Design review of the part built by this model. Coordinates are the model's own, in mm. Face numbers are marked on the shaded views. Coordinates: 2 decimals unless noted, no trailing zeros. Loops run counter-clockwise (first coordinate to the right, second up) from the corner with the lowest first, then second, coordinate; pieces in that order, holes last. Notation, with made-up numbers: M 33.5,19.5 L 79.5,19.5 A15 ccw 79.5,30.5 Z; hole C -22,-5 d7. An arc over 180 degrees is marked long. Write item = value, one per line. Start each with the question number.
```python
from build123d import *

# Parameters (mm, degrees)
SKETCH1_R                            = 5.08
BOSS_EXTRUDE1_DEPTH                  = 88.9
TAPPED_HOLE_FOR_4_40_HELICOIL1_D     = 3.048
TAPPED_HOLE_FOR_4_40_HELICOIL1_DEPTH = 8.128
TAPPED_HOLE_FOR_4_40_HELICOIL1_TIP   = 0.915711583
TAPPED_HOLE_FOR_4_40_HELICOIL2_D     = 3.048
TAPPED_HOLE_FOR_4_40_HELICOIL2_DEPTH = 8.128
TAPPED_HOLE_FOR_4_40_HELICOIL2_TIP   = 0.915711583
CUT_EXTRUDE1_DEPTH                   = 6.08
CUT_EXTRUDE1_DEPTH_BACK              = 6.08
TAPPED_HOLE_FOR_4_40_HELICOIL3_D     = 3.048


with BuildPart() as part:
    # Sketch1 → Boss-Extrude1 (new body)
    with BuildSketch(Plane(origin=(0, 0, 0), x_dir=(1, 0, 0), z_dir=(0, 1, 0))):
        Circle(SKETCH1_R)
    extrude(amount=BOSS_EXTRUDE1_DEPTH)

    # Tapped Hole for #4-40 Helicoil1
    with Locations(Plane(origin=(0, 88.9, 0), x_dir=(1, 0, 0), z_dir=(0, 1, 0))):
        with Locations((0, 0)):
            Hole(TAPPED_HOLE_FOR_4_40_HELICOIL1_D / 2, depth=TAPPED_HOLE_FOR_4_40_HELICOIL1_DEPTH)
            with Locations((0, 0, -(TAPPED_HOLE_FOR_4_40_HELICOIL1_DEPTH + TAPPED_HOLE_FOR_4_40_HELICOIL1_TIP / 2))):  # 118° drill point
                Cone(0, TAPPED_HOLE_FOR_4_40_HELICOIL1_D / 2, TAPPED_HOLE_FOR_4_40_HELICOIL1_TIP, mode=Mode.SUBTRACT)

    # Tapped Hole for #4-40 Helicoil2
    with Locations(Plane(origin=(0, 0, 0), x_dir=(-1, 0, 0), z_dir=(0, -1, 0))):
        with Locations((0, 0)):
            Hole(TAPPED_HOLE_FOR_4_40_HELICOIL2_D / 2, depth=TAPPED_HOLE_FOR_4_40_HELICOIL2_DEPTH)
            with Locations((0, 0, -(TAPPED_HOLE_FOR_4_40_HELICOIL2_DEPTH + TAPPED_HOLE_FOR_4_40_HELICOIL2_TIP / 2))):  # 118° drill point
                Cone(0, TAPPED_HOLE_FOR_4_40_HELICOIL2_D / 2, TAPPED_HOLE_FOR_4_40_HELICOIL2_TIP, mode=Mode.SUBTRACT)

    # Sketch8 → Cut-Extrude1 (cut, two sides)
    with BuildSketch(Plane.XY) as cut_extrude1_sk:
        with BuildLine():
            ThreePointArc((5.08, 80.400130206), (3.902618898, 78.44506403), (3.4925, 76.2))
            Line((3.4925, 76.2), (3.4925, 38.1))
            ThreePointArc((3.4925, 38.1), (3.902618898, 35.85493597), (5.08, 33.899869794))
            Line((5.08, 33.899869794), (5.08, 80.400130206))
        make_face()
    extrude(amount=CUT_EXTRUDE1_DEPTH, mode=Mode.SUBTRACT)
    extrude(cut_extrude1_sk.sketch, amount=-CUT_EXTRUDE1_DEPTH_BACK, mode=Mode.SUBTRACT)

    # Tapped Hole for #4-40 Helicoil3 (through all)
    with Locations(Plane(origin=(3.4925, 0, 0), x_dir=(0, 0, -1), z_dir=(1, 0, 0))):
        with Locations((0, 69.85), (0, 44.45)):
            Hole(TAPPED_HOLE_FOR_4_40_HELICOIL3_D / 2)


solid = part.part
```
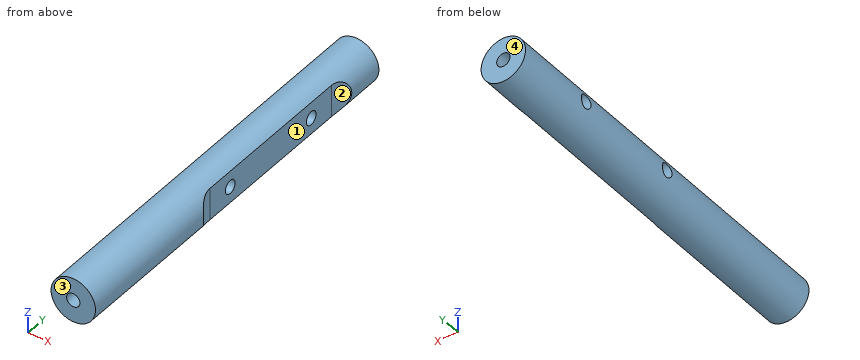
(1) To check wall thickness, follow L1, parallel to Z at x = 0, y = 2.25; L2, parallel to X at y = 17, z = -0.25; L3, parallel to X at y = 85, z = -0.5. State the ranges of each line that lie inside material, in increasing order.
(2) Take a section at A-A (y = 44.45). State the section outline as (x, z) points, plus the area to 3 significant figures.
(3) Take a section at C-C (y = 14). State the section outline as (x, z) points, plus the area to 3 significant figures.
(4) Insertion check: pin 1 (2.5 mm diameter, centred on x = 0, z = 0, fed in from +Y); pin 2 (2.5 mm diameter, centred on x = 0, z = 0, fed in from -Y); pin 3 (1.5 mm diameter, centred on x = -3, y = 28, fed in from +Z); pin 4 (2.5 mm diameter, centred on y = 69.85, z = 0, fed in from -X). Each pin has a flat end and moves straight along its axis. Give the tip position at first contact, or say it passes through.
(5) Take a section at D-D (x = 2.25). State the section outline as (y, z) points.
(6) Mouldability with a two-part tool opening along Y and no side actions: class the marked faces 1, 2, 3 and 4 as +Y half, -Y half, draft (parallel to the pull), parting line (faces both ways), or undercut.
(7) Take a section at B-B (z = -2.25). State the section outline as (x, y) points, plus the area to 3 significant figures.
Results list:
q1.L1 = -5.08 to -1.52, 1.52 to 5.08
q1.L2 = -5.07 to 5.07
q1.L3 = -5.06 to -1.44, 1.44 to 5.06
q2.outline = M -4.85,-1.52 A5.08 ccw 3.49,-3.69 L 3.49,-1.52 Z; M -4.85,1.52 L 3.49,1.52 L 3.49,3.69 A5.08 ccw Z
q2.area = 47.1 mm^2
q3.outline = C 0,0 d10.16
q3.area = 81.1 mm^2
q4.pin_1 = 80.61
q4.pin_2 = 8.29
q4.pin_3 = 4.55
q4.pin_4 = through
q5.outline = M 0,-4.55 L 88.9,-4.55 L 88.9,4.55 L 0,4.55 Z; hole C 44.45,0 d3.05; hole C 69.85,0 d3.05
q6.face_1 = undercut
q6.face_2 = undercut
q6.face_3 = -Y half
q6.face_4 = +Y half
q7.outline = M -4.55,0 L 4.55,0 L 4.55,34.58 A6.35 cw 3.49,38.1 L 3.49,76.2 A6.35 cw 4.55,79.72 L 4.55,88.9 L -4.55,88.9 Z
q7.area = 764 mm^2
